```python
from build123d import *

# Parameters (mm, degrees)
F0_R     = 2.5
F1_DEPTH = 25


with BuildPart() as f1:
    # F0 (on Front) → F1 (new body, symmetric)
    with BuildSketch(Plane.XZ):
        Polygon((9.631492, 20), (-9.631492, 20), (-21.641767, 4.939592), (-17.35535, -13.840429), (0, -22.198325), (17.35535, -13.840429), (21.641767, 4.939592), align=None)
        Circle(F0_R, mode=Mode.SUBTRACT)
        Circle(F0_R)
    extrude(amount=F1_DEPTH, both=True)


solid = f1.part
```
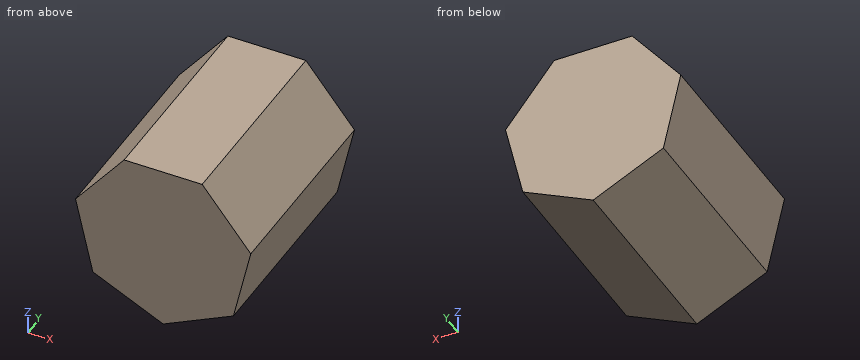
Design review of the part built by this model. Coordinates are the model's own, in mm. Round coordinates to 2 decimals unless told otherwise and drop trailing zeros. Write each loop counter-clockwise with the first axis right and the second up, starting at its lowest first coordinate (ties: lowest second). Pieces come first, ordered by that corner, then holes.
Item 1: Clearance check with flat-ended pins moving along their axes: pin 1 Ø1.5 at (x, y) = (14, 15) entering from +Z; pin 2 Ø8 at (y, z) = (-8, 8) entering from +X; pin 3 Ø12 at (y, z) = (1, -13.5) entering from -X. State where each tip first meets the part, or that it passes through.
Item 2: We need section B-B on z = -6. Write out the cut boundary in (x, y).
Item 3: For probe 1 along X at (y, z) = (-1.5, -11.5); probe 2 along Z at (x, y) = (-7.5, 5); probe 3 along Z at (x, y) = (-15, 14), list the stretches that pass through material, from the lowest coordinate up.
Item 4: We need section A-A on y = -5. Write out the cut boundary in (x, z).
Item 5: We need section C-C on x = -15. Write out the cut boundary in (y, z).
Returned:
1. pin 1: stops at z = 15.46
1. pin 2: stops at x = 21.64
1. pin 3: stops at x = -18.8
2. outline: (-19.14, -25) - (19.14, -25) - (19.14, 25) - (-19.14, 25) - close
3. probe 1: x = -17.89 to 17.89
3. probe 2: z = -18.59 to 20
3. probe 3: z = -14.97 to 13.27
4. outline: (-21.64, 4.94) - (-17.36, -13.84) - (0, -22.2) - (17.36, -13.84) - (21.64, 4.94) - (9.63, 20) - (-9.63, 20) - close
5. outline: (-25, -14.97) - (25, -14.97) - (25, 13.27) - (-25, 13.27) - close
